```python
from build123d import *

# Parameters (mm, degrees)
SKETCH1_R                   = 2
SKETCH1_W                   = 10
SKETCH1_H                   = 15
SKETCH1_W_2                 = 15
SKETCH1_H_2                 = 10
SKETCH1_W_3                 = 12
SKETCH1_H_3                 = 12
BOSS_EXTRUDE1_DEPTH         = 12
SKETCH2_R                   = 1
CUT_EXTRUDE1_DEPTH          = 12
ADVANCEDHOLE1_OUTLINE_R     = 2.25
ADVANCEDHOLE1_OUTLINE_R_2   = 2
ADVANCEDHOLE1_DEPTH         = 2.45
ADVANCEDHOLE1_DRAFT         = -45
ADVANCEDHOLE1_2_OUTLINE_R   = 2.25
ADVANCEDHOLE1_2_OUTLINE_R_2 = 2
ADVANCEDHOLE1_2_DEPTH       = 2.45
ADVANCEDHOLE1_2_DRAFT       = -45
ADVANCEDHOLE1_3_OUTLINE_R   = 2.25
ADVANCEDHOLE1_3_OUTLINE_R_2 = 2
ADVANCEDHOLE1_3_DEPTH       = 2.45
ADVANCEDHOLE1_3_DRAFT       = -45
ADVANCEDHOLE1_4_OUTLINE_R   = 2.25
ADVANCEDHOLE1_4_OUTLINE_R_2 = 2
ADVANCEDHOLE1_4_DEPTH       = 2.45
ADVANCEDHOLE1_4_DRAFT       = -45


# Read off the part's stored shape, not the designer's step: AdvancedHole1
with BuildPart() as part:
    # Sketch1 → Boss-Extrude1 (new body)
    with BuildSketch(Plane(origin=(0, 0, 0), x_dir=(1, 0, 0), z_dir=(0, 1, 0))):
        with BuildLine():
            Line((0, 1), (0, 190))
            ThreePointArc((0, 190), (6.540737726, 192.709262274), (9.25, 199.25))
            Line((9.25, 199.25), (10.25, 199.25))
            Line((10.25, 199.25), (198.25, 199.25))
            ThreePointArc((198.25, 199.25), (198.957106781, 198.957106781), (199.25, 198.25))
            Line((199.25, 198.25), (199.25, 155))
            ThreePointArc((199.25, 155), (198.957106781, 154.292893219), (198.25, 154))
            Line((198.25, 154), (95.25, 154))
            ThreePointArc((95.25, 154), (59.894660941, 139.355339059), (45.25, 104))
            Line((45.25, 104), (45.25, 1))
            ThreePointArc((45.25, 1), (44.957106781, 0.292893219), (44.25, 0))
            Line((44.25, 0), (1, 0))
            ThreePointArc((1, 0), (0.292893219, 0.292893219), (0, 1))
        make_face()
        with Locations(Location((60.75, 184, 0), (0, 0, 270))):
            Circle(SKETCH1_R, mode=Mode.SUBTRACT)
        with Locations(Location((154.75, 184, 0), (0, 0, 270))):
            Circle(SKETCH1_R, mode=Mode.SUBTRACT)
        with Locations(Location((15.25, 138.5, 0), (0, 0, 270))):
            Circle(SKETCH1_R, mode=Mode.SUBTRACT)
        with Locations(Location((15.25, 44.5, 0), (0, 0, 270))):
            Circle(SKETCH1_R, mode=Mode.SUBTRACT)
        with Locations((26.25, 91.5)):
            Rectangle(SKETCH1_W, SKETCH1_H, mode=Mode.SUBTRACT)
        with Locations((107.75, 173)):
            Rectangle(SKETCH1_W_2, SKETCH1_H_2, mode=Mode.SUBTRACT)
        with Locations((42.25, 184)):
            Rectangle(SKETCH1_W_3, SKETCH1_H_3, mode=Mode.SUBTRACT)
        with Locations((173.25, 184)):
            Rectangle(SKETCH1_W_3, SKETCH1_H_3, mode=Mode.SUBTRACT)
        with Locations((79.25, 184)):
            Rectangle(SKETCH1_W_3, SKETCH1_H_3, mode=Mode.SUBTRACT)
        with Locations((136.25, 184)):
            Rectangle(SKETCH1_W_3, SKETCH1_H_3, mode=Mode.SUBTRACT)
        with Locations((15.25, 120)):
            Rectangle(SKETCH1_W_3, SKETCH1_H_3, mode=Mode.SUBTRACT)
        with Locations((15.25, 26)):
            Rectangle(SKETCH1_W_3, SKETCH1_H_3, mode=Mode.SUBTRACT)
        with Locations((15.25, 63)):
            Rectangle(SKETCH1_W_3, SKETCH1_H_3, mode=Mode.SUBTRACT)
        with Locations((15.25, 157)):
            Rectangle(SKETCH1_W_3, SKETCH1_H_3, mode=Mode.SUBTRACT)
    extrude(amount=BOSS_EXTRUDE1_DEPTH)

    # Sketch2 → Cut-Extrude1 (cut)
    with BuildSketch(Plane(origin=(0, 0, 0), x_dir=(1, 0, 0), z_dir=(0, 1, 0))):
        with Locations((9.25, 151)):
            Circle(SKETCH2_R)
        with Locations((9.25, 163)):
            Circle(SKETCH2_R)
        with Locations((21.25, 163)):
            Circle(SKETCH2_R)
        with Locations((21.25, 151)):
            Circle(SKETCH2_R)
        with Locations((21.25, 126)):
            Circle(SKETCH2_R)
        with Locations((9.25, 114)):
            Circle(SKETCH2_R)
        with Locations((9.25, 126)):
            Circle(SKETCH2_R)
        with Locations((21.25, 114)):
            Circle(SKETCH2_R)
        with Locations((21.25, 69)):
            Circle(SKETCH2_R)
        with Locations((21.25, 57)):
            Circle(SKETCH2_R)
        with Locations((9.25, 57)):
            Circle(SKETCH2_R)
        with Locations((9.25, 69)):
            Circle(SKETCH2_R)
        with Locations((21.25, 32)):
            Circle(SKETCH2_R)
        with Locations((21.25, 20)):
            Circle(SKETCH2_R)
        with Locations((9.25, 20)):
            Circle(SKETCH2_R)
        with Locations((9.25, 32)):
            Circle(SKETCH2_R)
        with Locations((48.25, 178)):
            Circle(SKETCH2_R)
        with Locations((48.25, 190)):
            Circle(SKETCH2_R)
        with Locations((36.25, 190)):
            Circle(SKETCH2_R)
        with Locations((36.25, 178)):
            Circle(SKETCH2_R)
        with Locations((73.25, 178)):
            Circle(SKETCH2_R)
        with Locations((85.25, 178)):
            Circle(SKETCH2_R)
        with Locations((85.25, 190)):
            Circle(SKETCH2_R)
        with Locations((73.25, 190)):
            Circle(SKETCH2_R)
        with Locations((130.25, 178)):
            Circle(SKETCH2_R)
        with Locations((130.25, 190)):
            Circle(SKETCH2_R)
        with Locations((142.25, 190)):
            Circle(SKETCH2_R)
        with Locations((142.25, 178)):
            Circle(SKETCH2_R)
        with Locations((167.25, 178)):
            Circle(SKETCH2_R)
        with Locations((167.25, 190)):
            Circle(SKETCH2_R)
        with Locations((179.25, 190)):
            Circle(SKETCH2_R)
        with Locations((179.25, 178)):
            Circle(SKETCH2_R)
    extrude(amount=CUT_EXTRUDE1_DEPTH, mode=Mode.SUBTRACT)


with BuildPart() as advancedhole1_tool:
    # AdvancedHole1 outline → AdvancedHole1 (with draft: the straight prism first)
    with BuildSketch(Plane(origin=(0, 9.55, 0), x_dir=(1, 0, 0), z_dir=(0, 1, 0))):
        with Locations((154.75, 184)):
            Circle(ADVANCEDHOLE1_OUTLINE_R)
        with Locations((154.75, 184)):
            Circle(ADVANCEDHOLE1_OUTLINE_R_2, mode=Mode.SUBTRACT)
    extrude(amount=ADVANCEDHOLE1_DEPTH)
    # AdvancedHole1: the draft: its side faces are tilted about the plane it starts from
    advancedhole1_sides = [advancedhole1_tool.faces().sort_by_distance(p)[0] for p in [
        (152.5, 10.775, -184),
        (152.75, 10.775, -184),
    ]]
    draft(advancedhole1_sides, Plane(origin=(0, 9.55, 0), x_dir=(1, 0, 0), z_dir=(0, 1, 0)), ADVANCEDHOLE1_DRAFT)


with BuildPart() as part_1:
    add(part.part)

    # AdvancedHole1: cut by advancedhole1_tool
    add(advancedhole1_tool.part, mode=Mode.SUBTRACT)


with BuildPart() as advancedhole1_2_tool:
    # AdvancedHole1 2 outline → AdvancedHole1 2 (with draft: the straight prism first)
    with BuildSketch(Plane(origin=(0, 9.55, 0), x_dir=(1, 0, 0), z_dir=(0, 1, 0))):
        with Locations((60.75, 184)):
            Circle(ADVANCEDHOLE1_2_OUTLINE_R)
        with Locations((60.75, 184)):
            Circle(ADVANCEDHOLE1_2_OUTLINE_R_2, mode=Mode.SUBTRACT)
    extrude(amount=ADVANCEDHOLE1_2_DEPTH)
    # AdvancedHole1 2: the draft: its side faces are tilted about the plane it starts from
    advancedhole1_2_sides = [advancedhole1_2_tool.faces().sort_by_distance(p)[0] for p in [
        (58.5, 10.775, -184),
        (58.75, 10.775, -184),
    ]]
    draft(advancedhole1_2_sides, Plane(origin=(0, 9.55, 0), x_dir=(1, 0, 0), z_dir=(0, 1, 0)), ADVANCEDHOLE1_2_DRAFT)


with BuildPart() as part_2:
    add(part_1.part)

    # AdvancedHole1 2: cut by advancedhole1_2_tool
    add(advancedhole1_2_tool.part, mode=Mode.SUBTRACT)


with BuildPart() as advancedhole1_3_tool:
    # AdvancedHole1 3 outline → AdvancedHole1 3 (with draft: the straight prism first)
    with BuildSketch(Plane(origin=(0, 9.55, 0), x_dir=(1, 0, 0), z_dir=(0, 1, 0))):
        with Locations((15.25, 138.5)):
            Circle(ADVANCEDHOLE1_3_OUTLINE_R)
        with Locations((15.25, 138.5)):
            Circle(ADVANCEDHOLE1_3_OUTLINE_R_2, mode=Mode.SUBTRACT)
    extrude(amount=ADVANCEDHOLE1_3_DEPTH)
    # AdvancedHole1 3: the draft: its side faces are tilted about the plane it starts from
    advancedhole1_3_sides = [advancedhole1_3_tool.faces().sort_by_distance(p)[0] for p in [
        (13, 10.775, -138.5),
        (13.25, 10.775, -138.5),
    ]]
    draft(advancedhole1_3_sides, Plane(origin=(0, 9.55, 0), x_dir=(1, 0, 0), z_dir=(0, 1, 0)), ADVANCEDHOLE1_3_DRAFT)


with BuildPart() as part_3:
    add(part_2.part)

    # AdvancedHole1 3: cut by advancedhole1_3_tool
    add(advancedhole1_3_tool.part, mode=Mode.SUBTRACT)


with BuildPart() as advancedhole1_4_tool:
    # AdvancedHole1 4 outline → AdvancedHole1 4 (with draft: the straight prism first)
    with BuildSketch(Plane(origin=(0, 9.55, 0), x_dir=(1, 0, 0), z_dir=(0, 1, 0))):
        with Locations((15.25, 44.5)):
            Circle(ADVANCEDHOLE1_4_OUTLINE_R)
        with Locations((15.25, 44.5)):
            Circle(ADVANCEDHOLE1_4_OUTLINE_R_2, mode=Mode.SUBTRACT)
    extrude(amount=ADVANCEDHOLE1_4_DEPTH)
    # AdvancedHole1 4: the draft: its side faces are tilted about the plane it starts from
    advancedhole1_4_sides = [advancedhole1_4_tool.faces().sort_by_distance(p)[0] for p in [
        (13, 10.775, -44.5),
        (13.25, 10.775, -44.5),
    ]]
    draft(advancedhole1_4_sides, Plane(origin=(0, 9.55, 0), x_dir=(1, 0, 0), z_dir=(0, 1, 0)), ADVANCEDHOLE1_4_DRAFT)


with BuildPart() as part_4:
    add(part_3.part)

    # AdvancedHole1 4: cut by advancedhole1_4_tool
    add(advancedhole1_4_tool.part, mode=Mode.SUBTRACT)


solid = part_4.part
```
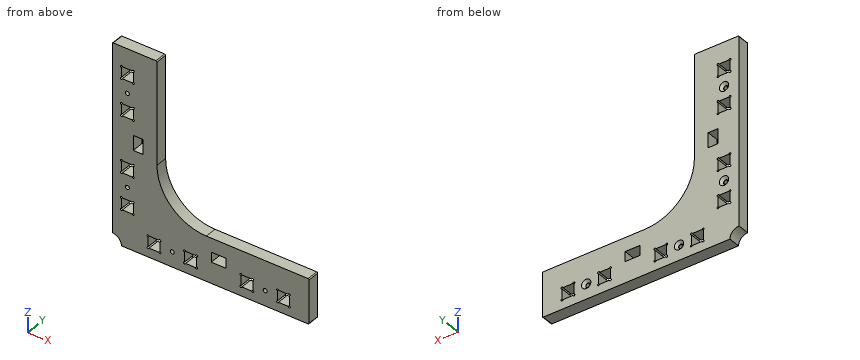
Geometry check sheet. Reference: the model listing, model coordinates, mm. Coordinates: 2 decimals unless noted, no trailing zeros. Loops run counter-clockwise (first coordinate to the right, second up) from the corner with the lowest first, then second, coordinate; pieces in that order, holes last. Notation, with made-up numbers: (7, 70) - (26, 70) arc R6 cw to (26, 79) - close; hole circle Ø2 at (32.5, -4.5). An arc over 180 degrees is marked (long way). One line per item, written item: value. Start each with the question number.
(1) Depth check by flat-ended pin: P1, Ø1.8, axis at x = 142.25, z = -178, coming from the +Y side; P2, Ø2, axis at y = 5.5, z = -123.5, coming from the +X side; P3, Ø3.5, axis at x = 110.5, y = 5.5, coming from the +Z side. Enter the tip coordinate at first touch or a pass-through.
(2) Material ranges on line 1 (X direction, y = 9, z = -181); line 2 (X direction, y = 4, z = -160); line 3 (Z direction, x = 137, y = 6.75), recorded low to high. Write a range as [from, to].
(3) Cross-section at B-B on y = 3.5. Count the separate pieces of the cut face and the enclosed holes in it, plus the area to 3 significant figures.
(4) Cross-section at A-A on x = 184.5. Enter the section's corners in (y, z), plus the area to 3 significant figures.
(5) Cross-section at C-C on z = -129.5. Enter the section's corners in (x, y).
Results below:
1. P1: passes through
1. P2: stops at x = 49.65
1. P3: stops at z = -154
2. line 1: x = [0, 36.25], [48.25, 73.25], [85.25, 130.25], [142.25, 167.25], [179.25, 199.25]
2. line 2: x = [0, 9.25], [21.25, 199.25]
2. line 3: z = [-199.25, -190], [-178, -154]
3. separate pieces: 1
3. enclosed holes: 14
3. area: 14,900 mm2
4. outline: (0, -199.25) - (12, -199.25) - (12, -154) - (0, -154) - close
4. area: 543 mm2
5. outline: (0, 0) - (52.24, 0) - (52.24, 12) - (0, 12) - close
